Can you work these out from the model? Positions are in its coordinate system, mm. Coordinates: 2 decimals unless noted, no trailing zeros. Answer as a JSON object with one key per item and string values.
from build123d import *
from build123d.topology import SkipClean

# Parameters (mm, degrees)
SKETCH3_R           = 33
SKETCH3_R_2         = 28
BOSS_EXTRUDE1_DEPTH = 35


with BuildPart() as part:
    # Sketch1 → Revolve1 (revolve)
    with SkipClean():  # the faces are left unmerged after this step: merging them gives an invalid solid
        with BuildSketch(Plane.XY):
            with BuildLine():
                Line((200, 0), (200, 42.32828037))
                add(Edge.make_bspline(
                    [(67.88595875, 19.569501359), (71.843085895, 20.404078353), (85.043129663, 23.124182603), (107.543506327, 27.445507457), (139.404169497, 33.021435572), (168.514660807, 37.655823826), (188.335942781, 40.630483181), (198.835243463, 42.159255501), (200, 42.32828037)],
                    knots=[0.116883244, 0.116883244, 0.116883244, 0.116883244, 0.116883244, 0.143539857, 0.205716573, 0.267893284, 0.330069995, 0.337827743, 0.337827743, 0.337827743, 0.337827743, 0.337827743], degree=4))
                ThreePointArc((67.88595875, 19.569501359), (84.611949981, 15.532965385), (92.013260114, 0))
                Line((92.013260114, 0), (200, 0))
            make_face()
            with BuildLine():
                ThreePointArc((92.013260114, 0), (84.611949981, 15.532965385), (67.88595875, 19.569501359))
                ThreePointArc((67.88595875, 19.569501359), (56.48029473, 12.598689867), (52.013260114, 0))
                Line((52.013260114, 0), (92.013260114, 0))
            make_face()
            with BuildLine():
                ThreePointArc((52.013260114, 0), (72.013260114, -20), (92.013260114, 0))
                Line((92.013260114, 0), (52.013260114, 0))
            make_face()
        revolve(axis=Axis((806.72, 0, 0), (-1, 0, 0)))
    add(part.part.scale(1), mode=Mode.REPLACE)  # the faces are merged on a copy

    # Sketch3 → Boss-Extrude1 (add)
    with BuildSketch(Plane(origin=(200, 0, 0), x_dir=(0, 0, -1), z_dir=(1, 0, 0))):
        Circle(SKETCH3_R)
        Circle(SKETCH3_R_2, mode=Mode.SUBTRACT)
    extrude(amount=BOSS_EXTRUDE1_DEPTH)


solid = part.part
Item 1: I'm going to push flat-ended pins straight in: pin 1 (3 mm diameter, centred on x = 213.5, z = 14, fed in from +Y); pin 2 (1.5 mm diameter, centred on x = 115.5, y = -19, fed in from -Z); pin 3 (2 mm diameter, centred on x = 173, z = 19, fed in from +Y). Where does each tip first touch, or does it pass through?
Answers follow:
{"pin 1": "stops at y = 30.54", "pin 2": "stops at z = -22.26", "pin 3": "stops at y = 33.82"}
Item 2: If we mould it in two halves opening along Y, with no side actions, what happens to faces 1 (the cylindrical face through (217.3, -12.6, -30.5)), 2 (the flat face through (235, -24, 15)), 3 (the flat face through (200, 0, 0)), 4 (the cylindrical face through (217.255, -10.724, -25.865))? For each: pulls with the +Y half, pulls with the -Y half, needs draft (parallel to the pull), parting line crosses it, or undercut.
Answers follow:
{"face 1": "parting line crosses it", "face 2": "needs draft", "face 3": "undercut", "face 4": "undercut"}
Item 3: Please list where these lines run through material, in increasing order: line 1 (Y direction, x = 221, z = 0); line 2 (Y direction, x = 218, z = 8.5); line 3 (Y direction, x = 184.5, z = -3).
Answers follow:
{"line 1": "y = -33 to -28, 28 to 33", "line 2": "y = -31.89 to -26.68, 26.68 to 31.89", "line 3": "y = -39.93 to 39.93"}
